Answer from the drawing. Dimensions are ordinates in mm from the lowest x, y and z of the part. A direction names the side the tool comes from. Give positions to 0.01 mm unless a question says otherwise; leave off trailing zeros. Order: outer loops, then holes, each group sorted by start corner. A loop starts at its lowest first (then second) coordinate and runs counter-clockwise, first axis right, second up.
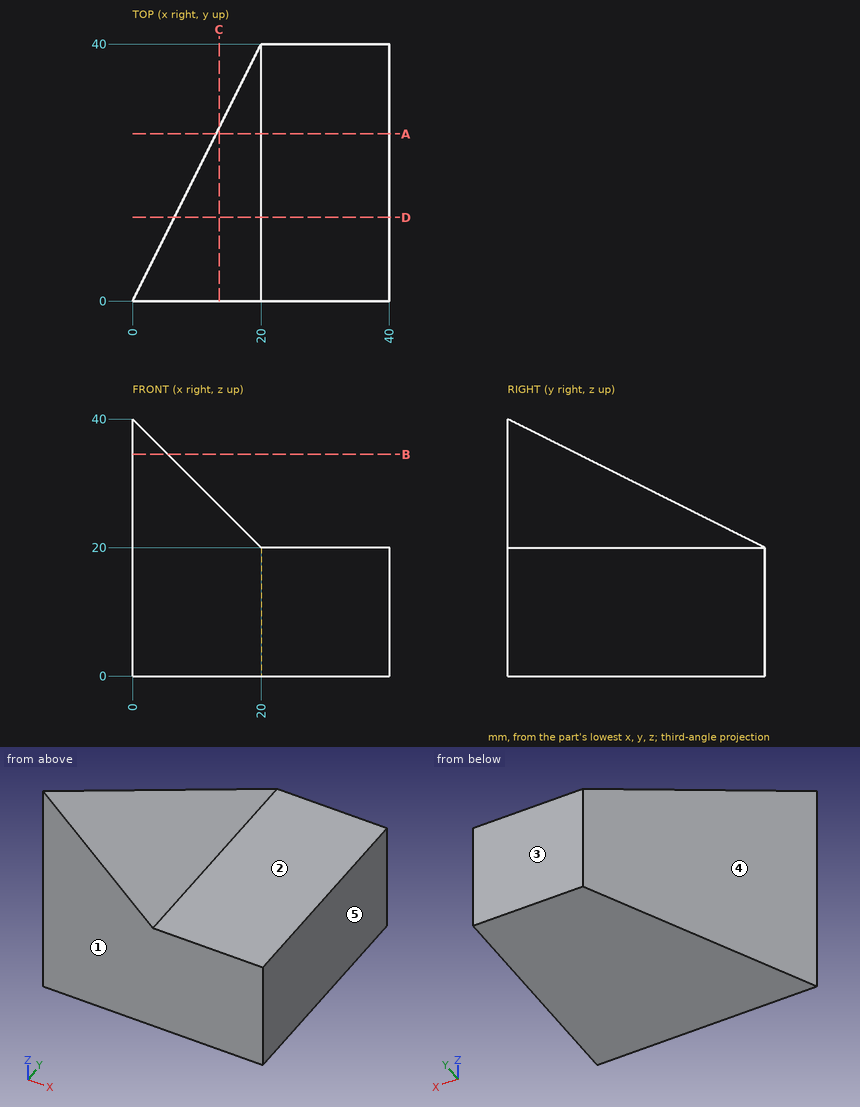
1) The part is cut by section B-B on z = 34.5. Determine the outline of the cut face in (x, y).
Final values:
outline: (0, 0) - (5.5, 0) - (5.5, 11) - close
2) A tool of negligible diameter and unlimited length cuts with its end or side. For the marked faces 1 and 2, from which of +Z, -Z, +X, -X, +Y, -Y can it reach the whole face along a straight path? Write none if from no direction.
Final values:
face 1: +Z, -Z, +X, -X, -Y
face 2: +Z, +X, +Y, -Y
3) The part is cut by section C-C on x = 13.5. Determine the outline of the cut face in (y, z), and give its area (4 significant figures).
Final values:
outline: (0, 0) - (27, 0) - (27, 26.5) - (0, 26.5) - close
area: 715.5 mm2
4) For a pull along X with two mould halves and no side action, classify the marked faces 3, 4 and 5 as released by +X, released by -X, zero draft, split by the parting line, or undercut.
Final values:
face 3: zero draft
face 4: released by -X
face 5: released by +X
5) Given pin 1 (5 mm diameter, centred on x = 24, y = 29.5, fed in from +Z); pin 2 (10 mm diameter, centred on y = 14.5, z = 17, fed in from -X); pin 3 (4 mm diameter, centred on x = 8.5, z = 21.5, fed in from +Y), each flat-ended and moving along its own axis, determine where each tip first touches the part or whether it passes through.
Final values:
pin 1: stops at z = 20
pin 2: stops at x = 4.75
pin 3: stops at y = 21
6) The part is cut by section A-A on y = 26. Determine the outline of the cut face in (x, z), and give its area (4 significant figures).
Final values:
outline: (13, 0) - (40, 0) - (40, 20) - (20, 20) - (13, 27) - close
area: 564.5 mm2
7) The part is cut by section D-D on y = 13. Determine the outline of the cut face in (x, z).
Final values:
outline: (6.5, 0) - (40, 0) - (40, 20) - (20, 20) - (6.5, 33.5) - close
8) Consider L1, parallel to Z at x = 33, y = 6.5; L2, parallel to Y at x = 4.5, z = 23.5; L3, parallel to X at y = 2, z = 4. Determine where each line is inside the solid, lowest interval first.
Final values:
L1: z = 0 to 20
L2: y = 0 to 9
L3: x = 1 to 40
